Part model, mm, in its own coordinate system. Face numbers are marked on the shaded views. A direction names the side the tool comes from. Give positions to 0.01 mm unless a question says otherwise; leave off trailing zeros. Write each loop counter-clockwise with the first axis right and the second up, starting at its lowest first coordinate (ties: lowest second). Pieces come first, ordered by that corner, then holes. Notation, with made-up numbers: M -3,31 L 1,31 A28 cw 1,52 Z; hole C -2,8.25 d11. An arc over 180 degrees is marked long. Answer as CSV lines item,"result". Start each with the question number.
Item 1: Band-saw the part on C-C, the plane z = 5.5. List the corners of the cut face in (x, y).
Item 2: Wall check: L1, parallel to Y at x = 0, z = 7.5; L2, parallel to Y at x = -1.75, z = -3.25; L3, parallel to Z at x = -7, y = 4. Give the ranges that are in metal, low to high. Write a range as from..to.
Item 3: 3-axis set-ups, long thin cutter, end or side, ignore diameter. For the marked faces 5, 6, 7, 8 and 9: which of +Z, -Z, +X, -X, +Y, -Y reach the whole face in a straight line?
Item 4: Band-saw the part on A-A, the plane z = -10. List the corners of the cut face in (x, y), then the cut area to 3 significant figures.
Item 5: Band-saw the part on B-B, the plane y = 0. List the corners of the cut face in (x, z), then the cut area to 3 significant figures.
Item 6: Pin check, flat tips, straight feed: pin 1 (0.5 mm diameter, centred on y = 0, z = -1, fed in from +X); pin 2 (3 mm diameter, centred on x = -5.5, z = -4, fed in from +Y); pin 3 (4.5 mm diameter, centred on x = 8.98, z = 5.5, fed in from -Y); pin 4 (3 mm diameter, centred on x = 8.98, z = 5.5, fed in from +Y). Stop position of each tip, or through.
Item 7: Two-plate mould, pull along Z, no slides. Class the marked faces 1, 2, 3 and 4: +Z half, -Z half, draft (parallel to the pull), parting line (faces both ways), or undercut.
from build123d import *

# Parameters (mm, degrees)
SKETCH1_R               = 15
SKETCH1_R_2             = 3
BOSS_EXTRUDE1_DEPTH     = 12.5
SKETCH2_R               = 15
CUT_EXTRUDE1_DEPTH      = 11
CUT_EXTRUDE2_DEPTH      = 12
CUT_EXTRUDE3_DEPTH      = 1.7
CUT_EXTRUDE4_DEPTH      = 25.622144504
CUT_EXTRUDE4_DEPTH_BACK = 25.622144504
SKETCH7_R               = 2
CUT_EXTRUDE5_START      = 4.85
SKETCH8_R               = 3.75
CUT_EXTRUDE5_DEPTH      = 21.299006117
FILLET1_R               = 2
FILLET2_R               = 1
CHAMFER1_SIZE           = 0.3


with BuildPart() as part:
    # Sketch1 → Boss-Extrude1 (new, symmetric)
    with BuildSketch(Plane.XY):
        Circle(SKETCH1_R)
        Circle(SKETCH1_R_2, mode=Mode.SUBTRACT)
    extrude(amount=BOSS_EXTRUDE1_DEPTH, both=True)

    # Sketch2 → Cut-Extrude1 (cut)
    with BuildSketch(Plane(origin=(0, 0, -12.5), x_dir=(-1, 0, 0), z_dir=(0, 0, -1))):
        with Locations((-16, 0)):
            Circle(SKETCH2_R)
        with Locations((16, 0)):
            Circle(SKETCH2_R)
    extrude(amount=-CUT_EXTRUDE1_DEPTH, mode=Mode.SUBTRACT)

    # Sketch3 → Cut-Extrude2 (cut)
    with BuildSketch(Plane(origin=(0, 0, -12.5), x_dir=(-1, 0, 0), z_dir=(0, 0, -1))):
        with BuildLine():
            Line((7.954715583, -0.85), (11, -0.85))
            Line((11, -0.85), (11, 0.85))
            Line((11, 0.85), (7.954715583, 0.85))
            ThreePointArc((7.954715583, 0.85), (-8, 0), (7.954715583, -0.85))
        make_face()
    extrude(amount=-CUT_EXTRUDE2_DEPTH, mode=Mode.SUBTRACT)

    # Sketch6 → Cut-Extrude3 (cut)
    with BuildSketch(Plane(origin=(0, -0.85, 0), x_dir=(1, 0, 0), z_dir=(0, 1, 0))):
        Polygon((-11, 0.5), (15, -25.5), (15, 0.5), (15, 1.5), (-11, 1.5), align=None)
    extrude(amount=CUT_EXTRUDE3_DEPTH, mode=Mode.SUBTRACT)

    # Sketch7 → Cut-Extrude4 (cut, two sides: drawn at the far end of the back side and taken through both)
    with BuildSketch(Plane(origin=(0, 0, 0), x_dir=(1, 0, 0), z_dir=(0, 1, 0)).offset(-CUT_EXTRUDE4_DEPTH_BACK)):
        with Locations(Location((8.975897302, -5.5, 0), (0, 0, 270))):
            Circle(SKETCH7_R)
    extrude(amount=CUT_EXTRUDE4_DEPTH + CUT_EXTRUDE4_DEPTH_BACK, mode=Mode.SUBTRACT)

    # Sketch8 → Cut-Extrude5 (cut, through all)
    with BuildSketch(Plane(origin=(0, -0.85, 0), x_dir=(1, 0, 0), z_dir=(0, 1, 0)).offset(CUT_EXTRUDE5_START)):
        with Locations((8.975897302, -5.5)):
            Circle(SKETCH8_R)
    extrude(amount=CUT_EXTRUDE5_DEPTH, mode=Mode.SUBTRACT)

    # Fillet1
    fillet1_edges = [part.edges().sort_by_distance(p)[0] for p in [
        (-15, 0, 12.5),
    ]]
    fillet(fillet1_edges, radius=FILLET1_R)

    # Fillet2
    fillet2_edges = [part.edges().sort_by_distance(p)[0] for p in [
        (5.160499055, -10.368472369, -12.5),
        (-5.160499055, 10.368472369, -12.5),
        (-5.160499055, -10.368472369, -12.5),
        (5.160499055, 10.368472369, -12.5),
        (0, 8, -12.5),
        (0, -8, -12.5),
    ]]
    fillet(fillet2_edges, radius=FILLET2_R)

    # Chamfer1
    chamfer1_edges = [part.edges().sort_by_distance(p)[0] for p in [
        (12.923271403, 7.615054579, -1.5),
        (-15, 0, -1.5),
        (12.923271403, -7.615054579, -1.5),
    ]]
    chamfer(chamfer1_edges, length=CHAMFER1_SIZE)


solid = part.part
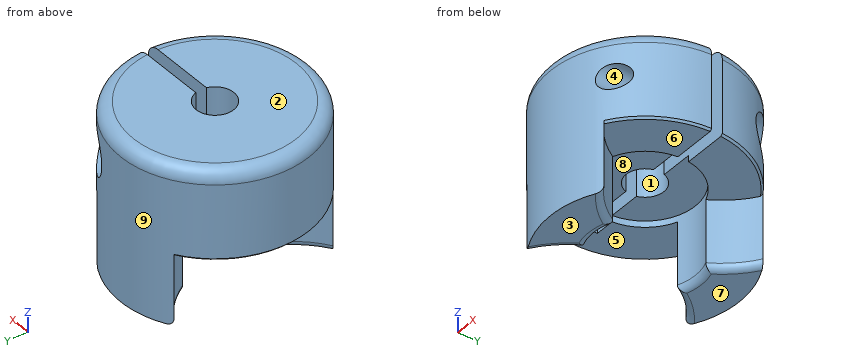
Output:
1,outline,"M -5,-0.85 L -5,0.85 L -2.88,0.85 A3 cw 2.88,0.85 L 6.98,0.85 L 6.98,4 L 5.23,4 L 5.23,14.06 A15 ccw long 6.98,-13.28 L 6.98,-0.85 L 2.88,-0.85 A3 cw -2.88,-0.85 Z; M 10.98,-10.22 A15 ccw 14.98,-0.85 L 10.98,-0.85 Z; M 10.98,0.85 L 14.98,0.85 A15 ccw 12.73,7.94 L 12.73,4 L 10.98,4 Z"
2,L1,"-15..-3, 3..15"
2,L2,"-14.9..-7.81, 7.81..14.9"
2,L3,"-1.5..12.5"
3,face 5,"-Z, -X"
3,face 6,"-Z, +X"
3,face 7,"-Z, +X, -X, +Y, -Y"
3,face 8,"-Z"
3,face 9,"+Z, -Z"
4,outline,"M -8,-12.69 A15 ccw 8,-12.69 A15 cw 2.97,-7.43 A8 cw -2.97,-7.43 A15 cw Z; M -8,12.69 A15 cw -2.97,7.43 A8 cw 2.97,7.43 A15 cw 8,12.69 A15 ccw Z"
4,area,"152 mm²"
5,outline,"M -15,-1.2 L -14.7,-1.5 L -11,-1.5 L -11,-0.5 L -3,7.5 L -3,12.5 L -13,12.5 A2 ccw -15,10.5 Z"
5,area,"127 mm²"
6,pin 1,"x = -11"
6,pin 2,"y = 14.46"
6,pin 3,"y = -13.41"
6,pin 4,"through"
7,face 1,"draft"
7,face 2,"+Z half"
7,face 3,"-Z half"
7,face 4,"undercut"
